Geometry check sheet. Reference: the model listing, model coordinates, mm. Give positions to 0.01 mm unless a question says otherwise; leave off trailing zeros. Loops run counter-clockwise (first coordinate to the right, second up) from the corner with the lowest first, then second, coordinate; pieces in that order, holes last. Notation, with made-up numbers: (-31, -38) -> (27, -38) arc R24 ccw to (27, -27) -> close; hole circle Ø11 at (50.25, 81). An arc over 180 degrees is marked (long way). Write item = value, one per line. Start each with the question number.
```python
from build123d import *

# Parameters (mm, degrees)
SKETCH1_W           = 888.64
SKETCH1_H           = 360
BOSS_EXTRUDE1_DEPTH = 2
SKETCH8_W           = 12
SKETCH8_H           = 264.038311476
CUT_EXTRUDE6_DEPTH  = 10
SKETCH9_R           = 2.5
SKETCH9_W           = 150
SKETCH9_H           = 150
CUT_EXTRUDE7_DEPTH  = 10


with BuildPart() as part:
    # Sketch1 → Boss-Extrude1 (new body)
    with BuildSketch(Plane(origin=(0, 0, 0), x_dir=(1, 0, 0), z_dir=(0, 1, 0))):
        with Locations((-18.597777778, 10.916666667)):
            Rectangle(SKETCH1_W, SKETCH1_H)
    extrude(amount=BOSS_EXTRUDE1_DEPTH)

    # Sketch8 → Cut-Extrude6 (cut)
    with BuildSketch(Plane(origin=(0, 2, 0), x_dir=(1, 0, 0), z_dir=(0, 1, 0))):
        with Locations((-433.323058676, 7.182390304)):
            Rectangle(SKETCH8_W, SKETCH8_H)
    extrude(amount=-CUT_EXTRUDE6_DEPTH, mode=Mode.SUBTRACT)

    # Sketch9 → Cut-Extrude7 (cut)
    with BuildSketch(Plane(origin=(0, 2, 0), x_dir=(1, 0, 0), z_dir=(0, 1, 0))):
        with Locations((223.018484234, 88.838711225)):
            Circle(SKETCH9_R)
        with Locations((383.018484234, 88.838711225)):
            Circle(SKETCH9_R)
        with Locations((383.018484234, -71.161288775)):
            Circle(SKETCH9_R)
        with Locations((223.018484234, -71.161288775)):
            Circle(SKETCH9_R)
        with Locations((303.018484234, 8.838711225)):
            Rectangle(SKETCH9_W, SKETCH9_H)
    extrude(amount=-CUT_EXTRUDE7_DEPTH, mode=Mode.SUBTRACT)


solid = part.part
```
1) Section check A-A (x = 300.5). Enter the section's corners in (y, z), plus the area to 3 significant figures.
2) Section check B-B (z = 36.5). Enter the section's corners in (x, y), plus the area to 3 significant figures.
3) Thickness scan on line 1 (X direction, y = 1.45, z = 37); line 2 (Z direction, x = 222.5, y = 0.4); line 3 (X direction, y = 0.6, z = 75). Record the ranges inside material, lowest first.
4) Section check C-C (y = 1.3). Enter the section's corners in (x, z), plus the area to 3 significant figures.
Check result:
q1.outline = (0, -190.92) -> (2, -190.92) -> (2, -83.84) -> (0, -83.84) -> close; (0, 66.16) -> (2, 66.16) -> (2, 169.08) -> (0, 169.08) -> close
q1.area = 420 mm2
q2.outline = (-462.92, 0) -> (-439.32, 0) -> (-439.32, 2) -> (-462.92, 2) -> close; (-427.32, 0) -> (228.02, 0) -> (228.02, 2) -> (-427.32, 2) -> close; (378.02, 0) -> (425.72, 0) -> (425.72, 2) -> (378.02, 2) -> close
q2.area = 1,450 mm2
q3.line_1 = -462.92 to -439.32, -427.32 to 228.02, 378.02 to 425.72
q3.line_2 = -190.92 to -91.28, -86.39 to 68.72, 73.61 to 169.08
q3.line_3 = -462.92 to -439.32, -427.32 to 425.72
q4.outline = (-462.92, -190.92) -> (425.72, -190.92) -> (425.72, 169.08) -> (-462.92, 169.08) -> close; hole (-439.32, -139.2) -> (-427.32, -139.2) -> (-427.32, 124.84) -> (-439.32, 124.84) -> close; hole circle Ø5 at (223.02, -88.84); hole circle Ø5 at (223.02, 71.16); hole (228.02, -83.84) -> (378.02, -83.84) -> (378.02, 66.16) -> (228.02, 66.16) -> close; hole circle Ø5 at (383.02, -88.84); hole circle Ø5 at (383.02, 71.16)
q4.area = 294,000 mm2
